Input: part model. Units: mm. Frame: model coordinates. A direction names the side the tool comes from. Coordinates: 2 decimals unless noted, no trailing zeros. Write each loop counter-clockwise with the first axis right and the second up, starting at its lowest first coordinate (ties: lowest second). Pieces come first, ordered by that corner, then holes. Notation, with made-up numbers: (83.25, -17.75) - (115.25, -17.75) arc R30 ccw to (115.25, 7.25) - close; hole circle Ø4 at (23.25, 35). An arc over 180 degrees is marked (long way). Put each result on its own line as item: value. Start each with the question number.
1. Cut plane B-B, the plane z = 16. Return loops of the section in (x, y).
2. Access query for faces 4 (the cylindrical face through (-77.535, -39.038, 28.613)), 5 (the flat face through (-12, -24, 77.609)). Directions: +Z, -Z, +X, -X, +Y, -Y. A direction counts if a zero-diameter tool reaches every point of the face in a straight line with its end or side. Return the directions, or none.
3. Pull-direction query (Z, two-part tool) for faces 1 (the cylindrical face through (47.49, -24.27, 73.33)), 2 (the flat face through (-80, -21, 36)), 3 (the cylindrical face through (-0.867, -2.465, 39.704)); classes: released by +Z, released by -Z, zero draft, split by the parting line, or undercut.
4. Cut plane C-C, the plane x = 12. Return loops of the section in (y, z).
5. Cut plane D-D, the plane x = 32. Return loops of the section in (y, z), and give its area (4 significant figures).
6. Pin query (flat end, axial travel): pin 1 (5 mm diameter, centred on x = -55, y = -38, fed in from -Z); pin 2 (3 mm diameter, centred on x = -15.5, z = 21, fed in from -Y); pin 3 (1 mm diameter, centred on x = 36.5, z = 17.5, fed in from +Y); pin 4 (1.5 mm diameter, centred on x = 39.5, y = -10.5, fed in from +Z). Return the tip coordinate at first contact, or that it passes through.
7. Cut plane A-A, the plane x = -38. Return loops of the section in (y, z).
8. Line query: line 1 (Y direction, x = 32, z = 80); line 2 (X direction, y = -33, z = 58.5); line 3 (Y direction, x = -30.5, z = 29). Output: solid intervals per line, ascending.
from build123d import *

# Parameters (mm, degrees)
F0_W     = 137
F0_H     = 73
F0_R     = 4
F1_DEPTH = 5
F3_DEPTH = 38
F5_R     = 2.25
F6_DEPTH = 137.001
F7_R     = 2.25
F8_DEPTH = 5
F9_R     = 15
F10_R    = 20


with BuildPart() as f1:
    # F0 (on Front) → F1 (new body)
    with BuildSketch(Plane.XZ):
        with Locations((-11.5, 46.109202)):
            Rectangle(F0_W, F0_H)
        with Locations((-38, 43.609202)):
            Circle(F0_R, mode=Mode.SUBTRACT)
        with Locations((0, 43.609202)):
            Circle(F0_R, mode=Mode.SUBTRACT)
        with Locations((38, 43.609202)):
            Circle(F0_R, mode=Mode.SUBTRACT)
    extrude(amount=F1_DEPTH)

    # F2 (on face) → F3 (join)
    with BuildSketch(Plane.XZ.offset(5)):
        Polygon((-80, 82.609202), (-80, 9.609202), (-75, 9.609202), (-75, 34.583051), (-75, 77.609202), (52, 77.609202), (52, 9.609202), (57, 9.609202), (57, 82.609202), align=None)
    extrude(amount=F3_DEPTH)

    # F5 (on face) → F6 (cut, through all)
    with BuildSketch(Plane(origin=(-80, 0, 0), x_dir=(0, -1, 0), z_dir=(-1, 0, 0))):
        with Locations((38, 57.609202)):
            Circle(F5_R)
        with Locations((38, 30.609202)):
            Circle(F5_R)
    extrude(amount=-F6_DEPTH, mode=Mode.SUBTRACT)

    # F7 (on face) → F8 (cut, through all)
    with BuildSketch(Plane.XY.offset(82.609202)):
        with Locations((-55, -38)):
            Circle(F7_R)
        with Locations((-11.5, -38)):
            Circle(F7_R)
        with Locations((32, -38)):
            Circle(F7_R)
    extrude(amount=-F8_DEPTH, mode=Mode.SUBTRACT)

    # F9
    f9_edges = [f1.edges().sort_by_distance(p)[0] for p in [
        (-75, -24, 77.609202),
        (52, -24, 77.609202),
    ]]
    fillet(f9_edges, radius=F9_R)

    # F10
    f10_edges = [f1.edges().sort_by_distance(p)[0] for p in [
        (-80, -21.5, 82.609202),
        (57, -21.5, 82.609202),
    ]]
    fillet(f10_edges, radius=F10_R)


solid = f1.part
Report:
1. outline: (-80, -43) - (-75, -43) - (-75, -5) - (52, -5) - (52, -43) - (57, -43) - (57, 0) - (-80, 0) - close
2. face 4: +X, -X
2. face 5: -Z, -Y
3. face 1: released by -Z
3. face 2: zero draft
3. face 3: undercut
4. outline: (-43, 77.61) - (-5, 77.61) - (-5, 9.61) - (0, 9.61) - (0, 82.61) - (-43, 82.61) - close
5. outline: (-43, 77.61) - (-40.25, 77.61) - (-40.25, 82.61) - (-43, 82.61) - close; (-35.75, 77.61) - (-5, 77.61) - (-5, 9.61) - (0, 9.61) - (0, 82.61) - (-35.75, 82.61) - close
5. area: 532.5 mm^2
6. pin 1: stops at z = 77.61
6. pin 2: stops at y = -5
6. pin 3: stops at y = 0
6. pin 4: stops at z = 82.53
7. outline: (-43, 77.61) - (-5, 77.61) - (-5, 47.61) - (0, 47.61) - (0, 82.61) - (-43, 82.61) - close; (-5, 9.61) - (0, 9.61) - (0, 39.61) - (-5, 39.61) - close
8. line 1: y = -43 to -40.25, -35.75 to 0
8. line 2: x = -80 to -75, 52 to 57
8. line 3: y = -5 to 0
